Check sheet for the modelled part. Datum: model origin and axes. Units: mm. Face numbers are marked on the shaded views. Give positions to 0.01 mm unless a question says otherwise; leave off trailing zeros. Write each loop counter-clockwise with the first axis right and the second up, starting at its lowest first coordinate (ties: lowest second). Pieces come first, ordered by that corner, then holes. Notation, with made-up numbers: (13.25, 1) -> (72.25, 1) arc R22 ccw to (72.25, 28) -> close; hole circle Ø9 at (46.5, -19). An arc over 180 degrees is marked (long way). Write each question's results on one line, items separated by ' | '. Start each with the question number.
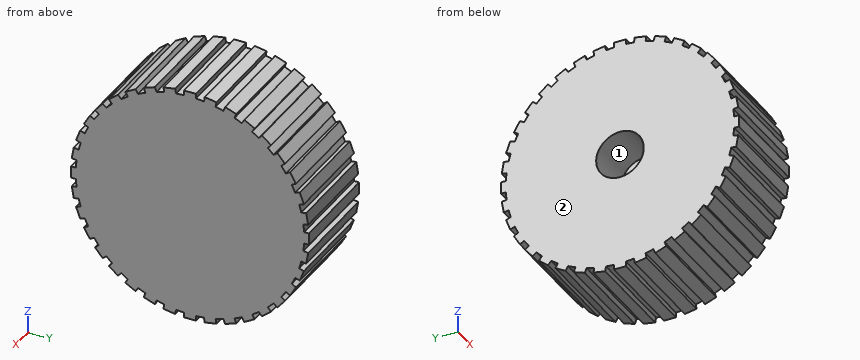
```python
from build123d import *

# Parameters (mm, degrees)
BOSS_EXTRUDE1_DEPTH = 200
SKETCH2_R           = 50
CUT_EXTRUDE1_DEPTH  = 100


with BuildPart() as part:
    # Sketch1 → Boss-Extrude1 (new body)
    with BuildSketch(Plane(origin=(0, 0, 0), x_dir=(0, 0, -1), z_dir=(1, 0, 0))):
        with BuildLine():
            Line((-12.5, 250), (12.5, 250))
            Line((12.5, 250), (12.5, 239.674258109))
            ThreePointArc((12.5, 239.674258109), (20.917378259, 239.086727542), (29.308901242, 238.203669804))
            Line((29.308901242, 238.203669804), (31.101947504, 248.372540474))
            Line((31.101947504, 248.372540474), (55.722141329, 244.031336032))
            Line((55.722141329, 244.031336032), (53.929095067, 233.862465362))
            ThreePointArc((53.929095067, 233.862465362), (62.116570825, 231.822198309), (70.22726635, 229.495383529))
            Line((70.22726635, 229.495383529), (73.758878072, 239.198406988))
            Line((73.758878072, 239.198406988), (97.251193591, 230.647903405))
            Line((97.251193591, 230.647903405), (93.71958187, 220.944879946))
            ThreePointArc((93.71958187, 220.944879946), (101.428382818, 217.513868889), (109.011811507, 213.813996155))
            Line((109.011811507, 213.813996155), (114.174682453, 222.756350946))
            Line((114.174682453, 222.756350946), (135.825317547, 210.256350946))
            Line((135.825317547, 210.256350946), (130.662446602, 201.313996155))
            ThreePointArc((130.662446602, 201.313996155), (137.658344724, 196.596490629), (144.484087934, 191.635978704))
            Line((144.484087934, 191.635978704), (151.121346883, 199.545955901))
            Line((151.121346883, 199.545955901), (170.272457961, 183.476265659))
            Line((170.272457961, 183.476265659), (163.635199012, 175.566288462))
            ThreePointArc((163.635199012, 175.566288462), (169.705627485, 169.705627485), (175.566288462, 163.635199012))
            Line((175.566288462, 163.635199012), (183.476265659, 170.272457961))
            Line((183.476265659, 170.272457961), (199.545955901, 151.121346883))
            Line((199.545955901, 151.121346883), (191.635978704, 144.484087934))
            ThreePointArc((191.635978704, 144.484087934), (196.596490629, 137.658344724), (201.313996155, 130.662446602))
            Line((201.313996155, 130.662446602), (210.256350946, 135.825317547))
            Line((210.256350946, 135.825317547), (222.756350946, 114.174682453))
            Line((222.756350946, 114.174682453), (213.813996155, 109.011811507))
            ThreePointArc((213.813996155, 109.011811507), (217.513868889, 101.428382818), (220.944879946, 93.71958187))
            Line((220.944879946, 93.71958187), (230.647903405, 97.251193591))
            Line((230.647903405, 97.251193591), (239.198406988, 73.758878072))
            Line((239.198406988, 73.758878072), (229.495383529, 70.22726635))
            ThreePointArc((229.495383529, 70.22726635), (231.822198309, 62.116570825), (233.862465362, 53.929095067))
            Line((233.862465362, 53.929095067), (244.031336032, 55.722141329))
            Line((244.031336032, 55.722141329), (248.372540474, 31.101947504))
            Line((248.372540474, 31.101947504), (238.203669804, 29.308901242))
            ThreePointArc((238.203669804, 29.308901242), (239.086727542, 20.917378259), (239.674258109, 12.5))
            Line((239.674258109, 12.5), (250, 12.5))
            Line((250, 12.5), (250, -12.5))
            Line((250, -12.5), (239.674258109, -12.5))
            ThreePointArc((239.674258109, -12.5), (239.086727542, -20.917378259), (238.203669804, -29.308901242))
            Line((238.203669804, -29.308901242), (248.372540474, -31.101947504))
            Line((248.372540474, -31.101947504), (244.031336032, -55.722141329))
            Line((244.031336032, -55.722141329), (233.862465362, -53.929095067))
            ThreePointArc((233.862465362, -53.929095067), (231.822198309, -62.116570825), (229.495383529, -70.22726635))
            Line((229.495383529, -70.22726635), (239.198406988, -73.758878072))
            Line((239.198406988, -73.758878072), (230.647903405, -97.251193591))
            Line((230.647903405, -97.251193591), (220.944879946, -93.71958187))
            ThreePointArc((220.944879946, -93.71958187), (217.513868889, -101.428382818), (213.813996155, -109.011811507))
            Line((213.813996155, -109.011811507), (222.756350946, -114.174682453))
            Line((222.756350946, -114.174682453), (210.256350946, -135.825317547))
            Line((210.256350946, -135.825317547), (201.313996155, -130.662446602))
            ThreePointArc((201.313996155, -130.662446602), (196.596490629, -137.658344724), (191.635978704, -144.484087934))
            Line((191.635978704, -144.484087934), (199.545955901, -151.121346883))
            Line((199.545955901, -151.121346883), (183.476265659, -170.272457961))
            Line((183.476265659, -170.272457961), (175.566288462, -163.635199012))
            ThreePointArc((175.566288462, -163.635199012), (169.705627485, -169.705627485), (163.635199012, -175.566288462))
            Line((163.635199012, -175.566288462), (170.272457961, -183.476265659))
            Line((170.272457961, -183.476265659), (151.121346883, -199.545955901))
            Line((151.121346883, -199.545955901), (144.484087934, -191.635978704))
            ThreePointArc((144.484087934, -191.635978704), (137.658344724, -196.596490629), (130.662446602, -201.313996155))
            Line((130.662446602, -201.313996155), (135.825317547, -210.256350946))
            Line((135.825317547, -210.256350946), (114.174682453, -222.756350946))
            Line((114.174682453, -222.756350946), (109.011811507, -213.813996155))
            ThreePointArc((109.011811507, -213.813996155), (101.428382818, -217.513868889), (93.71958187, -220.944879946))
            Line((93.71958187, -220.944879946), (97.251193591, -230.647903405))
            Line((97.251193591, -230.647903405), (73.758878072, -239.198406988))
            Line((73.758878072, -239.198406988), (70.22726635, -229.495383529))
            ThreePointArc((70.22726635, -229.495383529), (62.116570825, -231.822198309), (53.929095067, -233.862465362))
            Line((53.929095067, -233.862465362), (55.722141329, -244.031336032))
            Line((55.722141329, -244.031336032), (31.101947504, -248.372540474))
            Line((31.101947504, -248.372540474), (29.308901242, -238.203669804))
            ThreePointArc((29.308901242, -238.203669804), (20.917378259, -239.086727542), (12.5, -239.674258109))
            Line((12.5, -239.674258109), (12.5, -250))
            Line((12.5, -250), (-12.5, -250))
            Line((-12.5, -250), (-12.5, -239.674258109))
            ThreePointArc((-12.5, -239.674258109), (-20.917378259, -239.086727542), (-29.308901242, -238.203669804))
            Line((-29.308901242, -238.203669804), (-31.101947504, -248.372540474))
            Line((-31.101947504, -248.372540474), (-55.722141329, -244.031336032))
            Line((-55.722141329, -244.031336032), (-53.929095067, -233.862465362))
            ThreePointArc((-53.929095067, -233.862465362), (-62.116570825, -231.822198309), (-70.22726635, -229.495383529))
            Line((-70.22726635, -229.495383529), (-73.758878072, -239.198406988))
            Line((-73.758878072, -239.198406988), (-97.251193591, -230.647903405))
            Line((-97.251193591, -230.647903405), (-93.71958187, -220.944879946))
            ThreePointArc((-93.71958187, -220.944879946), (-101.428382818, -217.513868889), (-109.011811507, -213.813996155))
            Line((-109.011811507, -213.813996155), (-114.174682453, -222.756350946))
            Line((-114.174682453, -222.756350946), (-135.825317547, -210.256350946))
            Line((-135.825317547, -210.256350946), (-130.662446602, -201.313996155))
            ThreePointArc((-130.662446602, -201.313996155), (-137.658344724, -196.596490629), (-144.484087934, -191.635978704))
            Line((-144.484087934, -191.635978704), (-151.121346883, -199.545955901))
            Line((-151.121346883, -199.545955901), (-170.272457961, -183.476265659))
            Line((-170.272457961, -183.476265659), (-163.635199012, -175.566288462))
            ThreePointArc((-163.635199012, -175.566288462), (-169.705627485, -169.705627485), (-175.566288462, -163.635199012))
            Line((-175.566288462, -163.635199012), (-183.476265659, -170.272457961))
            Line((-183.476265659, -170.272457961), (-199.545955901, -151.121346883))
            Line((-199.545955901, -151.121346883), (-191.635978704, -144.484087934))
            ThreePointArc((-191.635978704, -144.484087934), (-196.596490629, -137.658344724), (-201.313996155, -130.662446602))
            Line((-201.313996155, -130.662446602), (-210.256350946, -135.825317547))
            Line((-210.256350946, -135.825317547), (-222.756350946, -114.174682453))
            Line((-222.756350946, -114.174682453), (-213.813996155, -109.011811507))
            ThreePointArc((-213.813996155, -109.011811507), (-217.513868889, -101.428382818), (-220.944879946, -93.71958187))
            Line((-220.944879946, -93.71958187), (-230.647903405, -97.251193591))
            Line((-230.647903405, -97.251193591), (-239.198406988, -73.758878072))
            Line((-239.198406988, -73.758878072), (-229.495383529, -70.22726635))
            ThreePointArc((-229.495383529, -70.22726635), (-231.822198309, -62.116570825), (-233.862465362, -53.929095067))
            Line((-233.862465362, -53.929095067), (-244.031336032, -55.722141329))
            Line((-244.031336032, -55.722141329), (-248.372540474, -31.101947504))
            Line((-248.372540474, -31.101947504), (-238.203669804, -29.308901242))
            ThreePointArc((-238.203669804, -29.308901242), (-239.086727542, -20.917378259), (-239.674258109, -12.5))
            Line((-239.674258109, -12.5), (-250, -12.5))
            Line((-250, -12.5), (-250, 12.5))
            Line((-250, 12.5), (-239.674258109, 12.5))
            ThreePointArc((-239.674258109, 12.5), (-239.086727542, 20.917378259), (-238.203669804, 29.308901242))
            Line((-238.203669804, 29.308901242), (-248.372540474, 31.101947504))
            Line((-248.372540474, 31.101947504), (-244.031336032, 55.722141329))
            Line((-244.031336032, 55.722141329), (-233.862465362, 53.929095067))
            ThreePointArc((-233.862465362, 53.929095067), (-231.822198309, 62.116570825), (-229.495383529, 70.22726635))
            Line((-229.495383529, 70.22726635), (-239.198406988, 73.758878072))
            Line((-239.198406988, 73.758878072), (-230.647903405, 97.251193591))
            Line((-230.647903405, 97.251193591), (-220.944879946, 93.71958187))
            ThreePointArc((-220.944879946, 93.71958187), (-217.513868889, 101.428382818), (-213.813996155, 109.011811507))
            Line((-213.813996155, 109.011811507), (-222.756350946, 114.174682453))
            Line((-222.756350946, 114.174682453), (-210.256350946, 135.825317547))
            Line((-210.256350946, 135.825317547), (-201.313996155, 130.662446602))
            ThreePointArc((-201.313996155, 130.662446602), (-196.596490629, 137.658344724), (-191.635978704, 144.484087934))
            Line((-191.635978704, 144.484087934), (-199.545955901, 151.121346883))
            Line((-199.545955901, 151.121346883), (-183.476265659, 170.272457961))
            Line((-183.476265659, 170.272457961), (-175.566288462, 163.635199012))
            ThreePointArc((-175.566288462, 163.635199012), (-169.705627485, 169.705627485), (-163.635199012, 175.566288462))
            Line((-163.635199012, 175.566288462), (-170.272457961, 183.476265659))
            Line((-170.272457961, 183.476265659), (-151.121346883, 199.545955901))
            Line((-151.121346883, 199.545955901), (-144.484087934, 191.635978704))
            ThreePointArc((-144.484087934, 191.635978704), (-137.658344724, 196.596490629), (-130.662446602, 201.313996155))
            Line((-130.662446602, 201.313996155), (-135.825317547, 210.256350946))
            Line((-135.825317547, 210.256350946), (-114.174682453, 222.756350946))
            Line((-114.174682453, 222.756350946), (-109.011811507, 213.813996155))
            ThreePointArc((-109.011811507, 213.813996155), (-101.428382818, 217.513868889), (-93.71958187, 220.944879946))
            Line((-93.71958187, 220.944879946), (-97.251193591, 230.647903405))
            Line((-97.251193591, 230.647903405), (-73.758878072, 239.198406988))
            Line((-73.758878072, 239.198406988), (-70.22726635, 229.495383529))
            ThreePointArc((-70.22726635, 229.495383529), (-62.116570825, 231.822198309), (-53.929095067, 233.862465362))
            Line((-53.929095067, 233.862465362), (-55.722141329, 244.031336032))
            Line((-55.722141329, 244.031336032), (-31.101947504, 248.372540474))
            Line((-31.101947504, 248.372540474), (-29.308901242, 238.203669804))
            ThreePointArc((-29.308901242, 238.203669804), (-20.917378259, 239.086727542), (-12.5, 239.674258109))
            Line((-12.5, 239.674258109), (-12.5, 250))
        make_face()
    extrude(amount=BOSS_EXTRUDE1_DEPTH)

    # Sketch2 → Cut-Extrude1 (cut)
    with BuildSketch(Plane.ZY):
        Circle(SKETCH2_R)
    extrude(amount=-CUT_EXTRUDE1_DEPTH, mode=Mode.SUBTRACT)


solid = part.part
```
Item 1: Mould release check, pull along Z, two halves, no side actions. Record for the marked faces 1 and 2: pulls with the +Z half, pulls with the -Z half, needs draft (parallel to the pull), parting line crosses it, or undercut.
Item 2: Depth check by flat-ended pin: pin 1 Ø8 at (x, y) = (167.5, 76.5) entering from -Z; pin 2 Ø5 at (x, z) = (100.5, 105) entering from -Y; pin 3 Ø1.5 at (x, y) = (67, 28.5) entering from -Z. Enter the tip coordinate at first touch or a pass-through.
Item 3: Thickness scan on probe 1 along Y at (x, z) = (39, 0); probe 2 along Y at (x, z) = (76, 132.5); probe 3 along Z at (x, y) = (84, 25.5). Record the ranges inside material, lowest first. Write a range as from..to.
Item 4: Section check A-A on z = 0. Record the boundary of the cut face in (x, y).
Check sheet entries:
1) face 1: undercut | face 2: needs draft
2) pin 1: stops at z = -239.2 | pin 2: stops at y = -217.01 | pin 3: stops at z = -238.39
3) probe 1: y = -250..-50, 50..250 | probe 2: y = -212.18..-204.5, -200.11..200.11, 204.5..212.18 | probe 3: z = -238.64..-43.01, 43.01..238.64
4) outline: (0, -250) -> (200, -250) -> (200, 250) -> (0, 250) -> (0, 50) -> (100, 50) -> (100, -50) -> (0, -50) -> close
